Geometry check sheet. Reference: the model listing, model coordinates, mm. Face numbers are marked on the shaded views. A direction names the side the tool comes from. Give positions to 0.01 mm unless a question says otherwise; leave off trailing zeros. Loops run counter-clockwise (first coordinate to the right, second up) from the corner with the lowest first, then second, coordinate; pieces in that order, holes last. Notation, with made-up numbers: (-26, 87) - (-15, 87) arc R26 cw to (-15, 126) - close; hole circle Ø1 at (-29.5, 56.25). An arc over 180 degrees is marked (long way). Use a Markdown table: item, result. Add a question column.
1. Cross-section at B-B on z = 0. Enter the section's corners in (x, y), and give its area (3 significant figures).
2. Set-up check for the marked faces 3 and 4: record each of +Z, -Z, +X, -X, +Y, -Y from which the full face is reachable in a straight line by a thin tool's end or side.
3. Draft check along X on the marked faces 1 and 2. Enter one of: pulls with the +X half, pulls with the -X half, needs draft (parallel to the pull), parting line crosses it, or undercut.
4. Material ranges on L1, parallel to Y at x = 6.25, z = 0.05; L2, parallel to Y at x = 15.5, z = -0.15; L3, parallel to X at y = 10.4, z = -0.05, recorded low to high.
5. Cross-section at A-A on x = 10.5. Enter the section's corners in (y, z), and give its area (3 significant figures).
from build123d import *

# Parameters (mm, degrees)
F1_R = 0.5


with BuildPart() as f2:
    # F2: sweep along a path in F0
    with BuildLine(Plane.XY) as f2_path:
        Line((0, 10), (1.5358983849, 10))
        Line((1.5358983849, 10), (5, 12))
        Line((5, 12), (10, 12))
    # F1 (on Right) → F2 (sweep)
    with BuildSketch(Plane.YZ):
        with Locations((10, 0)):
            Circle(F1_R)
    sweep(path=f2_path.line, transition=Transition.RIGHT)

    # F7: F2 across plane


with BuildPart() as f2_1:
    add(f2.part)
    add(f2.part.mirror(Plane.YZ.offset(10)))

    # F8: F2 across plane


with BuildPart() as f2_2:
    add(f2_1.part)
    add(f2_1.part.mirror(Plane.XZ.offset(-10)))


solid = f2_2.part
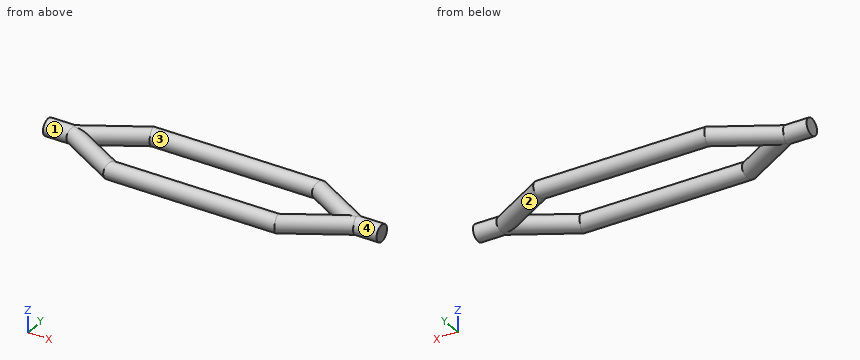
Values found:
| question | item | result |
|---|---|---|
| 1 | outline | (0, 9.5) - (1.4, 9.5) - (4.87, 7.5) - (15.13, 7.5) - (18.6, 9.5) - (20, 9.5) - (20, 10.5) - (18.6, 10.5) - (15.13, 12.5) - (4.87, 12.5) - (1.4, 10.5) - (0, 10.5) - close; hole (2.54, 10) - (5.13, 8.5) - (14.87, 8.5) - (17.46, 10) - (14.87, 11.5) - (5.13, 11.5) - close |
| 1 | area | 37.9 mm2 |
| 2 | face 3 | none |
| 2 | face 4 | +X |
| 3 | face 1 | needs draft |
| 3 | face 2 | undercut |
| 4 | L1 | y = 7.5 to 8.5, 11.5 to 12.5 |
| 4 | L2 | y = 7.74 to 8.84, 11.16 to 12.26 |
| 4 | L3 | x = 0 to 3.22, 16.78 to 20 |
| 5 | outline | circle Ø1 at (8, 0); circle Ø1 at (12, 0) |
| 5 | area | 1.57 mm2 |
